The listing builds one solid part. Answer for the finished solid, in the listing's coordinates (mm). Face numbers are marked on the shaded views. A direction names the side the tool comes from. Give positions to 0.01 mm unless a question says otherwise; leave off trailing zeros. Write each loop counter-clockwise with the first axis right and the second up, starting at its lowest first coordinate (ties: lowest second). Pieces come first, ordered by that corner, then holes. Notation, with made-up numbers: (18, 54.5) -> (43, 54.5) arc R21 cw to (43, 85.5) -> close; hole circle Ø1 at (59, 14.5). An arc over 180 degrees is marked (long way). Put each result on its own line as item: value. Start each with the question number.
1) Find the intervals of material crossed by line 1 along X through (y, z) = (1, -4.75); line 2 along Y through (x, z) = (11.5, -7.75); line 3 along Z through (x, y) = (-2, 8.5), in increasing order. Write a range as from..to.
2) For a pull along X with two mould halves and no side action, classify the marked faces 1, 2, 3 and 4 as released by +X, released by -X, zero draft, split by the parting line, or undercut.
3) A cutting plane is placed at D-D (z = -12). Write down the section's boundary in (x, y), then the cut area to 3 significant figures.
4) A cutting plane is placed at C-C (y = 3). Write down the section's boundary in (x, z), then the cut area to 3 significant figures.
5) For the marked faces 5, 6, 7 and 8, determine the directions among +Z, -Z, +X, -X, +Y, -Y from which every point of the face is accessible in a straight line to the end or side of a thin tool.
6) Flat-ended cylindrical pins translate along their axes: pin 1 Ø6 at (x, y) = (-3, 4.5) entering from -Z; pin 2 Ø5 at (x, y) = (2.5, 9.5) entering from +Z; pin 3 Ø2.5 at (x, z) = (-4, -10) entering from -Y. Find the tip coordinate at first contact, or state that the pin passes through.
7) A cutting plane is placed at A-A (z = -3). Write down the section's boundary in (x, y), then the cut area to 3 significant figures.
from build123d import *

# Parameters (mm, degrees)
SKETCH12_W               = 30
SKETCH12_H               = 15
BOSS_EXTRUDE4_DEPTH      = 10
CHAMFER1_SIZE            = 10
SKETCH14_W               = 24
SKETCH14_H               = 3
BOSS_EXTRUDE5_DEPTH      = 5
SKETCH15_W               = 30
SKETCH15_H               = 9
BOSS_EXTRUDE6_DEPTH      = 5
CUT_EXTRUDE10_DEPTH      = 37.431442464
CUT_EXTRUDE10_DEPTH_BACK = 37.431442464
CUT_EXTRUDE11_DEPTH      = 26.539185578
CUT_EXTRUDE11_DEPTH_BACK = 26.539185578
SKETCH18_W               = 26
SKETCH18_H               = 11


with BuildPart() as part:
    # Sketch12 → Boss-Extrude4 (new body)
    with BuildSketch(Plane(origin=(0, 0, 0), x_dir=(1, 0, 0), z_dir=(0, 1, 0))):
        Rectangle(SKETCH12_W, SKETCH12_H)
    extrude(amount=BOSS_EXTRUDE4_DEPTH)

    # Chamfer1
    chamfer1_edges = [part.edges().sort_by_distance(p)[0] for p in [
        (0, 10, 7.5),
    ]]
    chamfer(chamfer1_edges, length=CHAMFER1_SIZE - 0.0001)  # a hair under: the kernel refuses the full size

    # Sketch14 → Boss-Extrude5 (add)
    with BuildSketch(Plane(origin=(0, 0, -7.5), x_dir=(-1, 0, 0), z_dir=(0, 0, -1))):
        with Locations((0, 6.5)):
            Rectangle(SKETCH14_W, SKETCH14_H)
    extrude(amount=BOSS_EXTRUDE5_DEPTH)

    # Sketch15 → Boss-Extrude6 (add)
    with BuildSketch(Plane(origin=(0, 0, -12.5), x_dir=(-1, 0, 0), z_dir=(0, 0, -1))):
        with Locations((0, 6.5)):
            Rectangle(SKETCH15_W, SKETCH15_H)
    extrude(amount=BOSS_EXTRUDE6_DEPTH)

    # Sketch17 → Cut-Extrude10 (cut, two sides: drawn at the far end of the back side and taken through both)
    with BuildSketch(Plane.ZY.offset(15).offset(-CUT_EXTRUDE10_DEPTH_BACK)):
        Polygon((-12.5, 2), (-17.5, 11), (-17.5, 2), align=None)
    extrude(amount=CUT_EXTRUDE10_DEPTH + CUT_EXTRUDE10_DEPTH_BACK, mode=Mode.SUBTRACT)

    # Sketch18 → Cut-Extrude11 (cut, two sides: drawn at the far end of the back side and taken through both)
    with BuildSketch(Plane.XZ.offset(-CUT_EXTRUDE11_DEPTH_BACK)):
        Rectangle(SKETCH18_W, SKETCH18_H)
    extrude(amount=CUT_EXTRUDE11_DEPTH + CUT_EXTRUDE11_DEPTH_BACK, mode=Mode.SUBTRACT)


solid = part.part
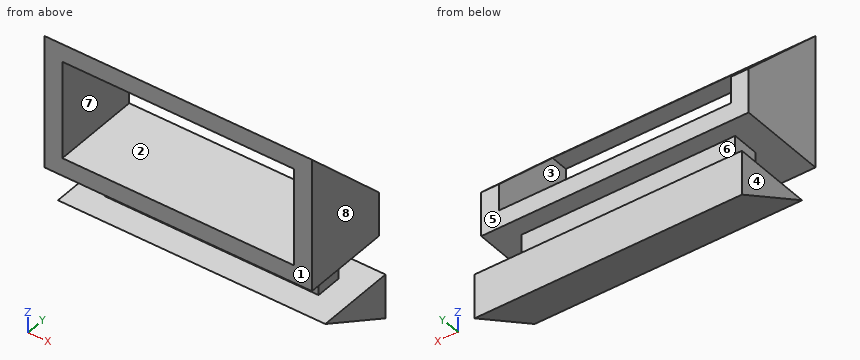
Reply:
1. line 1: x = -15..-13, 13..15
1. line 2: y = 5..8
1. line 3: z = -16.11..-12.5, -7.5..-5.5
2. face 1: zero draft
2. face 2: undercut
2. face 3: undercut
2. face 4: released by -X
3. outline: (-12, 5) -> (12, 5) -> (12, 8) -> (-12, 8) -> close
3. area: 72.0 mm2
4. outline: (-15, -13.06) -> (15, -13.06) -> (15, -12.5) -> (-15, -12.5) -> close; (-15, -7.5) -> (15, -7.5) -> (15, 4.5) -> (13, 4.5) -> (13, -5.5) -> (-13, -5.5) -> (-13, 4.5) -> (-15, 4.5) -> close
4. area: 117 mm2
5. face 5: +Z, +X, -X, +Y
5. face 6: +X, -X, +Y
5. face 7: +Y, -Y
5. face 8: +Z, -Z, +X, +Y, -Y
6. pin 1: stops at z = -15.56
6. pin 2: stops at z = -5.5
6. pin 3: stops at y = 5
7. outline: (-15, 0) -> (-13, 0) -> (-13, 10) -> (-15, 10) -> close; (13, 0) -> (15, 0) -> (15, 10) -> (13, 10) -> close
7. area: 40.0 mm2
